Work out the finished part from the listing and answer in its coordinate system (mm). Round coordinates to 2 decimals unless told otherwise and drop trailing zeros. Loops run counter-clockwise (first coordinate to the right, second up) from the corner with the lowest first, then second, coordinate; pieces in that order, holes last. Notation, with made-up numbers: (34, -35.75) - (45, -35.75) arc R10 cw to (45, -21.75) - close; hole circle Ø1 at (34.25, 6.5). An arc over 180 degrees is marked (long way). Return JSON: item names as keys, results as strings.
from build123d import *

# Parameters (mm, degrees)
F0_W      = 250.982642
F0_H      = 194.626228
F0_R      = 65.754774
F1_DEPTH  = 25
F1_FACE_W = 250.982642
F1_FACE_H = 194.626228
F1_FACE_R = 65.754774
F2_DEPTH  = 25


with BuildPart() as f1:
    # F0 (on Front) → F1 (new body)
    with BuildSketch(Plane.XZ):
        Rectangle(F0_W, F0_H)
        Circle(F0_R, mode=Mode.SUBTRACT)
    extrude(amount=F1_DEPTH)

    # F1_face (on face) → F2 (join)
    with BuildSketch(Plane(origin=(0, 0, 0), x_dir=(1, 0, 0), z_dir=(0, 1, 0))):
        Rectangle(F1_FACE_W, F1_FACE_H)
        Circle(F1_FACE_R, mode=Mode.SUBTRACT)
    extrude(amount=-F2_DEPTH)


solid = f1.part
1) Determine the mould class of faces 1 (the flat face through (-2, 0, 66)), 2 (the cylindrical face through (-14.254, -12.325, -64.191)), 3 (the flat face through (-2, -12, 97.313)) for opening direction Z: pulls with the +Z half, pulls with the -Z half, needs draft (parallel to the pull), parting line crosses it, or undercut.
Verdict:
{"face 1": "needs draft", "face 2": "undercut", "face 3": "pulls with the +Z half"}
2) Find the intervals of material crossed by L1, parallel to Z at x = 0, y = -8; L2, parallel to X at y = -23.5, z = 1; L3, parallel to X at y = -14.5, z = -16.5, in increasing order.
Verdict:
{"L1": "z = -97.31 to -65.75, 65.75 to 97.31", "L2": "x = -125.49 to -65.75, 65.75 to 125.49", "L3": "x = -125.49 to -63.65, 63.65 to 125.49"}
3) Section A-A (z = 0) is taken. Give the vertices of the cut face in (x, y), and give its area (3 significant figures).
Verdict:
{"outline": "(-125.49, -25) - (-65.75, -25) - (-65.75, 0) - (-125.49, 0) - close; (65.75, -25) - (125.49, -25) - (125.49, 0) - (65.75, 0) - close", "area": "2,990 mm2"}
4) A flat-ended cylindrical pin translates along its axis: pin 1 (1 mm diameter, centred on x = -1, z = -64, fed in from -Y). Find the tip coordinate at first contact, or state that the pin passes through.
Verdict:
{"pin 1": "passes through"}
5) Section C-C (y = -21.75) is taken. Give the vertices of the cut face in (x, z), and give its area (3 significant figures).
Verdict:
{"outline": "(-125.49, -97.31) - (125.49, -97.31) - (125.49, 97.31) - (-125.49, 97.31) - close; hole circle Ø131.51 at (0, 0)", "area": "35,300 mm2"}
6) Section B-B (x = 0) is taken. Give the vertices of the cut face in (y, z).
Verdict:
{"outline": "(-25, -97.31) - (0, -97.31) - (0, -65.75) - (-25, -65.75) - close; (-25, 65.75) - (0, 65.75) - (0, 97.31) - (-25, 97.31) - close"}
